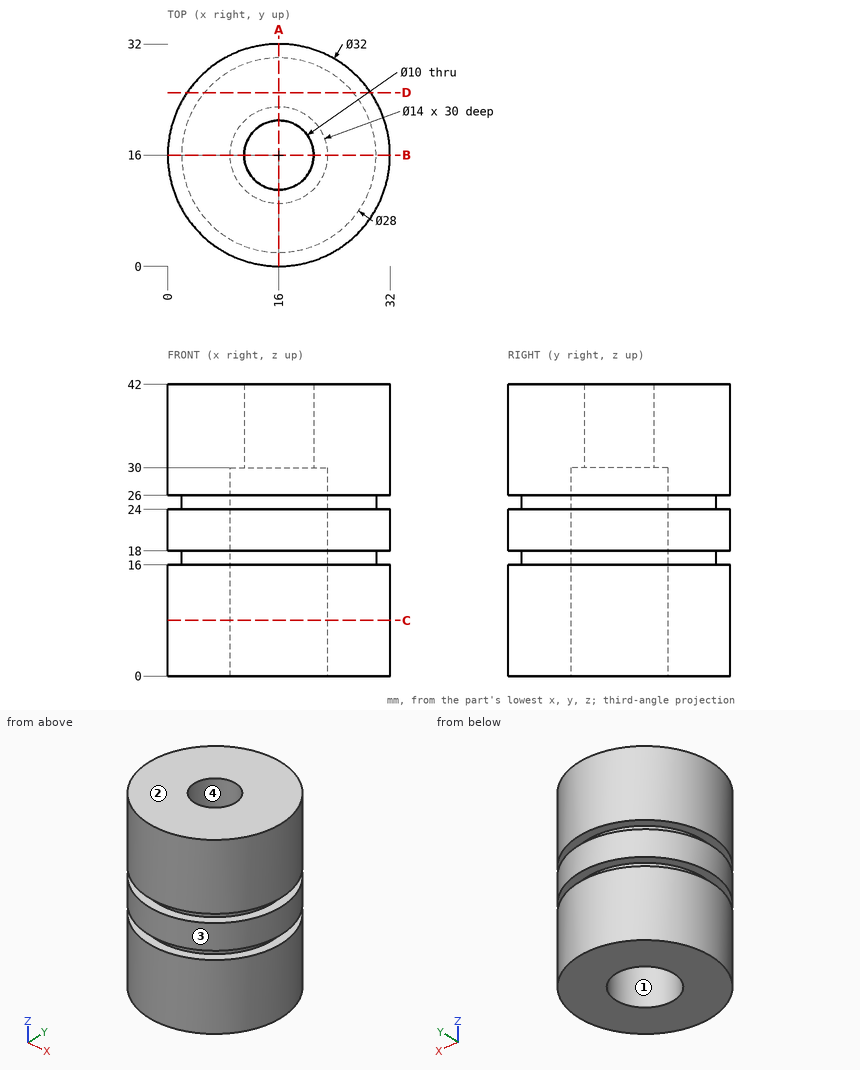
Input: dimensioned drawing with shaded views. Units: mm. Origin: part minimum x, y, z. Round coordinates to 2 decimals unless told otherwise and drop trailing zeros. Loops run counter-clockwise (first coordinate to the right, second up) from the corner with the lowest first, then second, coordinate; pieces in that order, holes last.
1) Section query A-A on x = 16. Return the cut outline in (y, z).
Ans:
outline: (0, 0) - (9, 0) - (9, 30) - (11, 30) - (11, 42) - (0, 42) - (0, 26) - (2, 26) - (2, 24) - (0, 24) - (0, 18) - (2, 18) - (2, 16) - (0, 16) - close; (21, 30) - (23, 30) - (23, 0) - (32, 0) - (32, 16) - (30, 16) - (30, 18) - (32, 18) - (32, 24) - (30, 24) - (30, 26) - (32, 26) - (32, 42) - (21, 42) - close
2) Pin query (flat end, axial travel): pin 1 (4 mm diameter, centred on x = 10, y = 18, fed in from -Z); pin 2 (6 mm diameter, centred on x = 24.5, z = 8, fed in from +Y) (3 decimals); pin 3 (4 mm diameter, centred on y = 14, z = 25, fed in from +X); pin 4 (3 mm diameter, centred on x = 7.5, z = 37, fed in from +Y). Return the tip coordinate at first contact, or that it passes through.
Ans:
pin 1: stops at z = 0
pin 2: stops at y = 31.025
pin 3: stops at x = 32
pin 4: stops at y = 30.39
3) Pull-direction query (Y, two-part tool) for the marked faces 1, 2, 3 and 4; classes: released by +Y, released by -Y, zero draft, split by the parting line, or undercut.
Ans:
face 1: undercut
face 2: zero draft
face 3: split by the parting line
face 4: undercut
4) Material intervals for line 1 (Z direction, x = 12.5, y = 1); line 2 (Y direction, x = 16, z = 35.25); line 3 (Y direction, x = 16, z = 14.5), sorted ascending.
Ans:
line 1: z = 0 to 16, 18 to 24, 26 to 42
line 2: y = 0 to 11, 21 to 32
line 3: y = 0 to 9, 23 to 32
5) Section query C-C on z = 8. Return the cut outline in (x, y).
Ans:
outline: circle Ø32 at (16, 16); hole circle Ø14 at (16, 16)
6) Section query D-D on y = 25. Return the cut outline in (x, z).
Ans:
outline: (2.77, 0) - (29.23, 0) - (29.23, 16) - (26.72, 16) - (26.72, 18) - (29.23, 18) - (29.23, 24) - (26.72, 24) - (26.72, 26) - (29.23, 26) - (29.23, 42) - (2.77, 42) - (2.77, 26) - (5.28, 26) - (5.28, 24) - (2.77, 24) - (2.77, 18) - (5.28, 18) - (5.28, 16) - (2.77, 16) - close
